Work out the finished part from the listing and answer in its coordinate system (mm). Give positions to 0.01 mm unless a question says otherwise; leave off trailing zeros. Order: outer loops, then holes, each group sorted by start corner. A loop starts at its lowest first (then second) coordinate and runs counter-clockwise, first axis right, second up. Notation, with made-up numbers: (-28, -38) - (22, -38) arc R19 cw to (22, -16) - close; hole circle Ø9 at (-33, 40.5). An arc over 180 degrees is marked (long way). Put each result on its own line as item: value.
```python
from build123d import *

# Parameters (mm, degrees)
SKETCH1_R             = 2.5
BOSS_EXTRUDE1_DEPTH   = 2
BOSS_EXTRUDE1_2_DEPTH = 2
BOSS_EXTRUDE2_DEPTH   = 10.1
SKETCH3_R             = 17.525
BOSS_EXTRUDE3_DEPTH   = 2
SKETCH4_R             = 2.75
CUT_EXTRUDE1_DEPTH    = 3
SKETCH2_3_W           = 10
SKETCH2_3_H           = 2
BOSS_EXTRUDE4_DEPTH   = 12.1
CUT_EXTRUDE2_REACH    = 77.098
SKETCH5_R             = 2.5
FILLET2_R             = 2
SKETCH6_R             = 2.75
CUT_EXTRUDE3_DEPTH    = 10


with BuildPart() as part:
    # Sketch1 → Boss-Extrude1 (new body)
    with BuildSketch(Plane.XY):
        with BuildLine():
            Line((-47.399346401, -23.901923789), (-44.399346401, -29.098076211))
            ThreePointArc((-44.399346401, -29.098076211), (-43.184933683, -30.029927864), (-41.667295593, -29.830127019))
            Line((-41.667295593, -29.830127019), (-36.47114317, -26.830127019))
            Line((-36.47114317, -26.830127019), (-41.47114317, -18.169872981))
            Line((-41.47114317, -18.169872981), (-46.667295593, -21.169872981))
            ThreePointArc((-46.667295593, -21.169872981), (-47.599147246, -22.384285698), (-47.399346401, -23.901923789))
        make_face()
        with Locations((-42.435244785, -24.5)):
            Circle(SKETCH1_R, mode=Mode.SUBTRACT)
    extrude(amount=BOSS_EXTRUDE1_DEPTH)



with BuildPart() as body_2:
    # Sketch1 → Boss-Extrude1 2 (new body)
    with BuildSketch(Plane.XY):
        with BuildLine():
            Line((41.667295593, -29.830127019), (36.47114317, -26.830127019))
            Line((36.47114317, -26.830127019), (41.47114317, -18.169872981))
            Line((41.47114317, -18.169872981), (46.667295593, -21.169872981))
            ThreePointArc((46.667295593, -21.169872981), (47.599147246, -22.384285698), (47.399346401, -23.901923789))
            Line((47.399346401, -23.901923789), (44.399346401, -29.098076211))
            ThreePointArc((44.399346401, -29.098076211), (43.184933683, -30.029927864), (41.667295593, -29.830127019))
        make_face()
        with Locations((42.435244785, -24.5)):
            Circle(SKETCH1_R, mode=Mode.SUBTRACT)
    extrude(amount=BOSS_EXTRUDE1_2_DEPTH)


with BuildPart() as part_1:
    add(part.part)

    add(body_2.part)  # Boss-Extrude2 merges body 2
    # Sketch2 → Boss-Extrude2 (add)
    with BuildSketch(Plane.XY.offset(2)):
        Polygon((41.47114317, -18.169872981), (36.47114317, -26.830127019), (34.739092363, -25.830127019), (39.739092363, -17.169872981), align=None)
        Polygon((-34.739092363, -25.830127019), (-39.739092363, -17.169872981), (-41.47114317, -18.169872981), (-36.47114317, -26.830127019), align=None)
    extrude(amount=-BOSS_EXTRUDE2_DEPTH)

    # Sketch3 → Boss-Extrude3 (add)
    with BuildSketch(Plane(origin=(0, 0, -8.1), x_dir=(-1, 0, 0), z_dir=(0, 0, -1))):
        with BuildLine():
            Line((-41.47114317, -18.169872981), (-36.47114317, -26.830127019))
            Line((-36.47114317, -26.830127019), (-13.845311828, -13.767097203))
            ThreePointArc((-13.845311828, -13.767097203), (0, -19.525), (13.845311828, -13.767097203))
            Line((13.845311828, -13.767097203), (36.47114317, -26.830127019))
            Line((36.47114317, -26.830127019), (41.47114317, -18.169872981))
            Line((41.47114317, -18.169872981), (18.845311828, -5.106843165))
            ThreePointArc((18.845311828, -5.106843165), (16.909146009, 9.7625), (5, 18.873940368))
            Line((5, 18.873940368), (5, 45))
            Line((5, 45), (-5, 45))
            Line((-5, 45), (-5, 18.873940368))
            ThreePointArc((-5, 18.873940368), (-16.909146009, 9.7625), (-18.845311828, -5.106843165))
            Line((-18.845311828, -5.106843165), (-41.47114317, -18.169872981))
        make_face()
        Circle(SKETCH3_R, mode=Mode.SUBTRACT)
    extrude(amount=BOSS_EXTRUDE3_DEPTH)

    # Sketch4 → Cut-Extrude1 (cut, through all)
    with BuildSketch(Plane.XY.offset(-8.1)):
        with Locations((0, 32.5)):
            Circle(SKETCH4_R)
    extrude(amount=-CUT_EXTRUDE1_DEPTH, mode=Mode.SUBTRACT)

    # Sketch2<3> → Boss-Extrude4 (add)
    with BuildSketch(Plane.XY.offset(2)):
        with Locations((0, 44)):
            Rectangle(SKETCH2_3_W, SKETCH2_3_H)
    extrude(amount=-BOSS_EXTRUDE4_DEPTH)

    # Sketch5 → Cut-Extrude2 (cut, up to next)
    with BuildSketch(Plane(origin=(0, 45, 0), x_dir=(1, 0, 0), z_dir=(0, 1, 0)), mode=Mode.PRIVATE) as cut_extrude2_sk1:
        with Locations((0, 2)):
            Circle(SKETCH5_R)
    cut_extrude2_tool1 = extrude(cut_extrude2_sk1.sketch, amount=-CUT_EXTRUDE2_REACH, mode=Mode.PRIVATE) & part_1.part
    add(cut_extrude2_tool1.solids().sort_by_distance((0, 45, -2))[0], mode=Mode.SUBTRACT)

    # Fillet2
    fillet2_edges = [part_1.edges().sort_by_distance(p)[0] for p in [
        (-37.239092363, -21.5, 2),
        (38.97114317, -22.5, -10.1),
        (-38.97114317, -22.5, -10.1),
        (0, 45, -10.1),
        (37.239092363, -21.5, 2),
        (5, 44, 2),
        (-5, 44, 2),
    ]]
    fillet(fillet2_edges, radius=FILLET2_R)

    # Sketch6 → Cut-Extrude3 (cut)
    with BuildSketch(Plane.XY.offset(-8.1)):
        with Locations((0, 32.5)):
            Circle(SKETCH6_R)
        with Locations((28.145825623, -16.25)):
            Circle(SKETCH6_R)
        with Locations((-28.145825623, -16.25)):
            Circle(SKETCH6_R)
    extrude(amount=-CUT_EXTRUDE3_DEPTH, mode=Mode.SUBTRACT)


solid = part_1.part
```
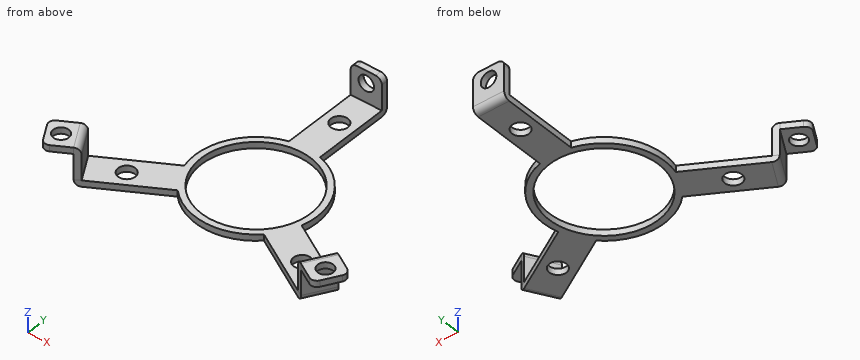
(1) Given pin 1 (5.5 mm diameter, centred on x = 42.5, y = -24.5, fed in from -Z); pin 2 (3 mm diameter, centred on x = 14.5, y = -17, fed in from -Z); pin 3 (6 mm diameter, centred on x = -14.5, z = -8, fed in from +Y); pin 4 (5 mm diameter, centred on y = 38.5, z = -6, fed in from -X), each flat-ended and moving along its own axis, determine where each tip first touches the part or whether it passes through.
Geometry check:
pin 1: stops at z = 0
pin 2: passes through
pin 3: stops at y = 15.78
pin 4: stops at x = -5
(2) Section A-A, the plane y = 32.5 is taken. Write down the section's boundary in (x, z), then the cut area to 3 significant figures.
Geometry check:
outline: (-5, -10.1) - (-2.75, -10.1) - (-2.75, -8.1) - (-5, -8.1) - close; (2.75, -10.1) - (5, -10.1) - (5, -8.1) - (2.75, -8.1) - close
area: 9.00 mm²
(3) Section C-C, the plane z = -2 is taken. Write down the section's boundary in (x, y), then the cut area to 3 significant figures.
Geometry check:
outline: (-41.47, -18.17) - (-36.47, -26.83) - (-34.74, -25.83) - (-39.74, -17.17) - close; (-5, 43) - (-2.5, 43) - (-2.5, 45) - (-5, 45) - close; (2.5, 43) - (5, 43) - (5, 45) - (2.5, 45) - close; (34.74, -25.83) - (36.47, -26.83) - (41.47, -18.17) - (39.74, -17.17) - close
area: 50.0 mm²
(4) Section B-B, the plane x = 0 is taken. Write down the section's boundary in (y, z) (3 decimals), then the cut area to 3 significant figures.
Geometry check:
outline: (-19.525, -10.1) - (-17.525, -10.1) - (-17.525, -8.1) - (-19.525, -8.1) - close; (17.525, -10.1) - (29.75, -10.1) - (29.75, -8.1) - (17.525, -8.1) - close; (35.25, -10.1) - (43, -10.1) arc R2 ccw to (45, -8.1) - (45, -4.5) - (43, -4.5) - (43, -8.1) - (35.25, -8.1) - close; (43, 0.5) - (45, 0.5) - (45, 2) - (43, 2) - close
area: 57.3 mm²
(5) Section D-D, the plane y = 0 is taken. Write down the section's boundary in (x, z) (3 decimals), then the cut area to 3 significant figures.
Geometry check:
outline: (-19.525, -10.1) - (-17.525, -10.1) - (-17.525, -8.1) - (-19.525, -8.1) - close; (17.525, -10.1) - (19.525, -10.1) - (19.525, -8.1) - (17.525, -8.1) - close
area: 8.00 mm²
(6) Straight lines are drawn through the part: line 1 (Z direction, x = 20, y = -15); line 2 (Y direction, x = -8.5, z = -8.5); line 3 (X direction, y = 11.5, z = -9). For each, find the intervals that lie inside material, in ascending order.
Geometry check:
line 1: z = -10.1 to -8.1
line 2: y = -17.58 to -15.33, 15.33 to 17.58
line 3: x = -15.78 to -13.22, 13.22 to 15.78
